Verification items for the finished model (mm, model axes). A direction names the side the tool comes from. Give positions to 0.01 mm unless a question says otherwise; leave off trailing zeros. Write each loop counter-clockwise with the first axis right and the second up, starting at its lowest first coordinate (ties: lowest second). Pieces come first, ordered by that corner, then holes. Notation, with made-up numbers: (25, -34.75) -> (72, -34.75) arc R30 ccw to (72, 3.25) -> close; hole circle Ø7 at (39.5, 61). An arc over 180 degrees is marked (long way). Use one line per item in the form item = value. Start each with the question number.
(1) Set-up check for faces 1 (the face through (50.751, -78.748, 163.752)), 2 (the face through (-1, -0.8, -1)): record each of +Z, -Z, +X, -X, +Y, -Y from which the full face is reachable in a straight line by a thin tool's end or side.
(2) Section check B-B, the plane y = -191.5. Record the cut outline in (x, z).
(3) Section check C-C, the plane z = 198.5. Record the cut outline in (x, y).
(4) Section check D-D, the plane x = -64.5. Record the cut outline in (y, z), plus the area to 3 significant figures.
(5) Depth check by flat-ended pin: pin 1 Ø22.5 at (x, z) = (23.5, 16.5) entering from -Y; pin 2 Ø6 at (x, y) = (15, -85) entering from +Z; pin 3 Ø8 at (x, z) = (-27.5, 156) entering from -Y. Enter the tip coordinate at first touch or a pass-through.
(6) Scan lines: L1, parallel to Y at x = 81, z = 25; L2, parallel to Z at x = 69.5, y = -13; L3, parallel to Z at x = 78, y = -157. Record each from-to range of solid material in increasing order.
(7) Section check A-A, the plane x = -11.5. Record the cut outline in (y, z), plus the area to 3 significant figures.
from build123d import *

# Parameters (mm, degrees)
SKETCH1_W                    = 180
SKETCH1_H                    = 75
BASE_FLANGE1_DEPTH           = 0.8
EDGE_FLANGE1_STRIP_CUT_DEPTH = 180
EDGE_FLANGE1_DEPTH           = 180
CUT_EXTRUDE1_DEPTH           = 10
TAB1_DEPTH                   = 0.8


# Sheet-metal steps are written as plain solids
with BuildPart() as part:
    # Sketch1 → Base-Flange1 (new body)
    with BuildSketch(Plane(origin=(0, 0, 0), x_dir=(1, 0, 0), z_dir=(0, 1, 0))):
        Rectangle(SKETCH1_W, SKETCH1_H)
    extrude(amount=-BASE_FLANGE1_DEPTH)

    # Edge-Flange1 strip (across the edge) → Edge-Flange1 strip cut (cut)
    with BuildSketch(Plane(origin=(90, -0.8, 37.5), x_dir=(0, -0.8480480961564291, -0.5299192642332), z_dir=(-1, 0, 0))):
        Polygon((-3.100489422, 3.452156347), (-0.556876954, -0.618474514), (0.121561523, -0.194539103), (-2.422050945, 3.876091759), align=None)
    extrude(amount=EDGE_FLANGE1_STRIP_CUT_DEPTH, mode=Mode.SUBTRACT)

    # Edge-Flange1 section (across the edge) → Edge-Flange1 (add)
    with BuildSketch(Plane(origin=(90, -0.8, 37.5), x_dir=(0, -0.8480480961564291, -0.5299192642332), z_dir=(-1, 0, 0))):
        with BuildLine():
            Line((-0.8, 0.229396309), (-0.8, 302.770603691))
            Line((-0.8, 302.770603691), (0, 302.770603691))
            Line((0, 302.770603691), (0, 0.229396309))
            ThreePointArc((0, 0.229396309), (0.030990643, 0.008886424), (0.121561523, -0.194539103))
            Line((0.121561523, -0.194539103), (-0.556876954, -0.618474514))
            ThreePointArc((-0.556876954, -0.618474514), (-0.738018714, -0.211623461), (-0.8, 0.229396309))
        make_face()
    extrude(amount=EDGE_FLANGE1_DEPTH)

    # Sketch5 → Cut-Extrude1 (cut)
    with BuildSketch(Plane(origin=(0, 16.955478386, 10.594958791), x_dir=(1, 0, 0), z_dir=(0, 0.8480480961564291, 0.5299192642332))):
        Polygon((-90, -32.455135326), (11.580249487, -360.607900661), (-238.910363798, -331.986176437), align=None)
    extrude(amount=-CUT_EXTRUDE1_DEPTH, mode=Mode.SUBTRACT)

    # Sketch6 → Tab1 (add)
    with BuildSketch(Plane(origin=(0, 16.955478386, 10.594958791), x_dir=(1, 0, 0), z_dir=(0, 0.8480480961564291, 0.5299192642332001))):
        Polygon((3.65214794, -334.996342709), (195.49906109, -420.380554221), (195.49906109, -348.383732857), (90, -334.996342709), align=None)
    extrude(amount=-TAB1_DEPTH)


solid = part.part
Completed:
q1.face_1 = +Z, +X, -X, +Y
q1.face_2 = -Z, +X, -X, -Y
q2.outline = (131.94, 342.68) -> (195.5, 342.68) -> (195.5, 344.19) -> (134.81, 344.19) -> close
q3.outline = (-31.46, -100.46) -> (-31.3, -101.4) -> (90, -101.4) -> (90, -100.46) -> close
q4.outline = (-44.57, 107.55) -> (-0.92, 37.69) arc R0.8 cw to (-0.8, 37.27) -> (-0.8, -37.5) -> (0, -37.5) -> (0, 37.27) arc R1.6 ccw to (-0.24, 38.12) -> (-43.9, 107.98) -> close
q4.area = 126 mm²
q5.pin_1 = -0.8
q5.pin_2 = 178.56
q5.pin_3 = -77.35
q6.L1 = -0.8 to 0
q6.L2 = 57.02 to 58.53
q6.L3 = 287.47 to 288.98
q7.outline = (-135.31, 252.75) -> (-0.92, 37.69) arc R0.8 cw to (-0.8, 37.27) -> (-0.8, -37.5) -> (0, -37.5) -> (0, 37.27) arc R1.6 ccw to (-0.24, 38.12) -> (-134.63, 253.18) -> close
q7.area = 263 mm²
